```python
from build123d import *

# Parameters (mm, degrees)
SKETCH1_W           = 76.2
SKETCH1_H           = 76.2
BOSS_EXTRUDE1_DEPTH = 88.9
SKETCH2_R           = 5.25
CUT_EXTRUDE1_DEPTH  = 300
SKETCH3_W           = 76.2
SKETCH3_H           = 63.5
CUT_EXTRUDE2_DEPTH  = 5
CUT_EXTRUDE5_DEPTH  = 140.7


with BuildPart() as part:
    # Sketch1 → Boss-Extrude1 (new body)
    with BuildSketch(Plane(origin=(0, 0, 0), x_dir=(1, 0, 0), z_dir=(0, 1, 0))):
        with Locations((38.1, 38.1)):
            Rectangle(SKETCH1_W, SKETCH1_H)
    extrude(amount=BOSS_EXTRUDE1_DEPTH)

    # Sketch2 → Cut-Extrude1 (cut)
    with BuildSketch(Plane.XY):
        with Locations((38.1, 57.15)):
            Circle(SKETCH2_R)
    extrude(amount=-CUT_EXTRUDE1_DEPTH, mode=Mode.SUBTRACT)

    # Sketch3 → Cut-Extrude2 (cut)
    with BuildSketch(Plane.XY):
        with Locations((38.1, 57.15)):
            Rectangle(SKETCH3_W, SKETCH3_H)
    extrude(amount=-CUT_EXTRUDE2_DEPTH, mode=Mode.SUBTRACT)

    # Sketch5 → Cut-Extrude5 (cut, through all)
    with BuildSketch(Plane(origin=(0, 88.9, 0), x_dir=(1, 0, 0), z_dir=(0, 1, 0))):
        Polygon((0, 76.2), (0, 30.4), (45.8, 76.2), align=None)
    extrude(amount=-CUT_EXTRUDE5_DEPTH, mode=Mode.SUBTRACT)


solid = part.part
```
Work out the finished part from the listing and answer in its coordinate system (mm). A direction names the side the tool comes from. Round coordinates to 2 decimals unless told otherwise and drop trailing zeros. Write each loop counter-clockwise with the first axis right and the second up, starting at its lowest first coordinate (ties: lowest second). Pieces come first, ordered by that corner, then holes. Notation, with made-up numbers: (-27.5, 38) -> (10.5, 38) arc R21 cw to (10.5, 50) -> close; hole circle Ø4 at (-29.75, 25.5). An arc over 180 degrees is marked (long way). Write each question's results on one line, items separated by ' | '.
1) The part is cut by section B-B (x = 38.1). Write down the section's boundary in (y, z).
Findings:
outline: (0, -68.5) -> (51.9, -68.5) -> (51.9, -5) -> (25.4, -5) -> (25.4, 0) -> (0, 0) -> close; (62.4, -68.5) -> (88.9, -68.5) -> (88.9, -5) -> (62.4, -5) -> close
2) For a pull along Y with two mould halves and no side action, classify faces 3 (the flat face through (46, 88.9, -33)), 4 (the flat face through (38, 65, -5)), 5 (the cylindrical face through (43.108, 58.727, -38.894)) as +Y half, -Y half, draft (parallel to the pull), parting line (faces both ways), or undercut.
Findings:
face 3: +Y half | face 4: draft | face 5: undercut
3) The part is cut by section C-C (z = -62.5). Write down the section's boundary in (x, y).
Findings:
outline: (32.1, 0) -> (76.2, 0) -> (76.2, 88.9) -> (32.1, 88.9) -> close; hole circle Ø10.5 at (38.1, 57.15)
4) Flat-ended cylindrical pins translate along their axes: pin 1 (12 mm diameter, centred on x = 38.1, y = 57.15, fed in from +Z); pin 2 (10 mm diameter, centred on y = 13, z = -57.5, fed in from -X); pin 3 (1 mm diameter, centred on x = 51.5, z = -41.5, fed in from -Y); pin 4 (1.5 mm diameter, centred on x = 26.5, z = -1.5, fed in from +Y). Find the tip coordinate at first contact, or state that the pin passes through.
Findings:
pin 1: stops at z = -5 | pin 2: stops at x = 22.1 | pin 3: stops at y = 0 | pin 4: stops at y = 25.4
5) Consider line 1 along X through (y, z) = (57, -20); line 2 along X through (y, z) = (57, -43); line 3 along Z through (x, y) = (59, 44.5). Determine where each line is inside the solid, lowest interval first. Write a range as [from, to].
Findings:
line 1: x = [0, 32.85], [43.35, 76.2] | line 2: x = [12.6, 32.85], [43.35, 76.2] | line 3: z = [-76.2, -5]
6) Which of the six approach directions +Z, -Z, +X, -X, +Y, -Y give full straight-line access (tool end or side, diameter ignored) to faces 1 (the flat face through (76.2, 44, -38)), 2 (the flat face through (38, 25.4, -2))?
Findings:
face 1: +Z, -Z, +X, +Y, -Y | face 2: +Z, +X, -X, +Y
7) The part is cut by section A-A (y = 57.15). Write down the section's boundary in (x, z), and give its area (3 significant figures).
Findings:
outline: (0, -30.4) -> (32.85, -63.25) -> (32.85, -5) -> (0, -5) -> close; (43.35, -73.75) -> (45.8, -76.2) -> (76.2, -76.2) -> (76.2, -5) -> (43.35, -5) -> close | area: 3,710 mm²
8) The part is cut by section D-D (x = 8.5). Write down the section's boundary in (y, z).
Findings:
outline: (0, -38.9) -> (88.9, -38.9) -> (88.9, -5) -> (25.4, -5) -> (25.4, 0) -> (0, 0) -> close
